from build123d import *

# Parameters (mm, degrees)
SKETCH1_W             = 80
SKETCH1_H             = 40
SKETCH1_R             = 2.25
BOSS_EXTRUDE1_DEPTH   = 5
BOSS_EXTRUDE1_2_DEPTH = 5
SKETCH2_W             = 80
SKETCH2_H             = 5
BOSS_EXTRUDE2_DEPTH   = 108.62
SKETCH3_W             = 43.85
SKETCH3_H             = 74
BOSS_EXTRUDE3_DEPTH   = 5
SKETCH5_W             = 29.85
SKETCH5_H             = 50
CUT_EXTRUDE2_DEPTH    = 10
CUT_EXTRUDE1_REACH    = 146.412
SKETCH4_R             = 1.3
FILLET1_R             = 3
FILLET2_R             = 3
SKETCH9_R             = 2.65
SKETCH9_R_2           = 1.05
BOSS_EXTRUDE5_DEPTH   = 4.75
SKETCH10_W            = 12
SKETCH10_H            = 6.8
CUT_EXTRUDE4_DEPTH    = 8
SKETCH11_W            = 80
SKETCH11_H            = 5
BOSS_EXTRUDE6_DEPTH   = 8
CUT_EXTRUDE5_REACH    = 167.987


with BuildPart() as part:
    # Sketch1 → Boss-Extrude1 (new body)
    with BuildSketch(Plane(origin=(0, 0, 0), x_dir=(1, 0, 0), z_dir=(0, 1, 0))):
        with Locations((0, 52)):
            Rectangle(SKETCH1_W, SKETCH1_H)
        with Locations(Location((-30.625, 53.044055982, 0), (0, 0, 270))):
            Circle(SKETCH1_R, mode=Mode.SUBTRACT)
        with Locations(Location((30.625, 53.044055982, 0), (0, 0, 90))):
            Circle(SKETCH1_R, mode=Mode.SUBTRACT)
    extrude(amount=BOSS_EXTRUDE1_DEPTH)



with BuildPart() as body_2:
    # Sketch1 → Boss-Extrude1 2 (new body)
    with BuildSketch(Plane(origin=(0, 0, 0), x_dir=(1, 0, 0), z_dir=(0, 1, 0))):
        with Locations((0, -52)):
            Rectangle(SKETCH1_W, SKETCH1_H)
        with Locations(Location((30.625, -53.044055982, 0), (0, 0, 270))):
            Circle(SKETCH1_R, mode=Mode.SUBTRACT)
        with Locations(Location((-30.625, -53.044055982, 0), (0, 0, 90))):
            Circle(SKETCH1_R, mode=Mode.SUBTRACT)
    extrude(amount=BOSS_EXTRUDE1_2_DEPTH)


with BuildPart() as part_1:
    add(part.part)

    add(body_2.part)  # Boss-Extrude2 merges body 2
    # Sketch2 → Boss-Extrude2 (add)
    with BuildSketch(Plane(origin=(0, 5, 0), x_dir=(1, 0, 0), z_dir=(0, 1, 0))):
        with Locations((0, 34.5)):
            Rectangle(SKETCH2_W, SKETCH2_H)
        with Locations((0, -34.5)):
            Rectangle(SKETCH2_W, SKETCH2_H)
    extrude(amount=BOSS_EXTRUDE2_DEPTH)

    # Sketch3 → Boss-Extrude3 (add)
    with BuildSketch(Plane(origin=(0, 113.62, 0), x_dir=(1, 0, 0), z_dir=(0, 1, 0))):
        with Locations((-3.925, 0)):
            Rectangle(SKETCH3_W, SKETCH3_H)
    extrude(amount=BOSS_EXTRUDE3_DEPTH)

    # Sketch5 → Cut-Extrude2 (cut)
    with BuildSketch(Plane.XZ.offset(-113.62)):
        with Locations((-3.925, 0)):
            Rectangle(SKETCH5_W, SKETCH5_H)
    extrude(amount=-CUT_EXTRUDE2_DEPTH, mode=Mode.SUBTRACT)

    # Sketch4 → Cut-Extrude1 (cut, up to next)
    with BuildSketch(Plane(origin=(0, 118.62, 0), x_dir=(1, 0, 0), z_dir=(0, 1, 0)), mode=Mode.PRIVATE) as cut_extrude1_sk1:
        with Locations(Location((-23, 20, 0), (0, 0, 270))):
            Circle(SKETCH4_R)
    cut_extrude1_tool1 = extrude(cut_extrude1_sk1.sketch, amount=-CUT_EXTRUDE1_REACH, mode=Mode.PRIVATE) & part_1.part
    # Sketch4 → Cut-Extrude1 (cut, up to next)
    with BuildSketch(Plane(origin=(0, 118.62, 0), x_dir=(1, 0, 0), z_dir=(0, 1, 0)), mode=Mode.PRIVATE) as cut_extrude1_sk2:
        with Locations(Location((15, 20, 0), (0, 0, 270))):
            Circle(SKETCH4_R)
    cut_extrude1_tool2 = extrude(cut_extrude1_sk2.sketch, amount=-CUT_EXTRUDE1_REACH, mode=Mode.PRIVATE) & part_1.part
    # Sketch4 → Cut-Extrude1 (cut, up to next)
    with BuildSketch(Plane(origin=(0, 118.62, 0), x_dir=(1, 0, 0), z_dir=(0, 1, 0)), mode=Mode.PRIVATE) as cut_extrude1_sk3:
        with Locations(Location((15, -20, 0), (0, 0, 270))):
            Circle(SKETCH4_R)
    cut_extrude1_tool3 = extrude(cut_extrude1_sk3.sketch, amount=-CUT_EXTRUDE1_REACH, mode=Mode.PRIVATE) & part_1.part
    # Sketch4 → Cut-Extrude1 (cut, up to next)
    with BuildSketch(Plane(origin=(0, 118.62, 0), x_dir=(1, 0, 0), z_dir=(0, 1, 0)), mode=Mode.PRIVATE) as cut_extrude1_sk4:
        with Locations(Location((-23, -20, 0), (0, 0, 270))):
            Circle(SKETCH4_R)
    cut_extrude1_tool4 = extrude(cut_extrude1_sk4.sketch, amount=-CUT_EXTRUDE1_REACH, mode=Mode.PRIVATE) & part_1.part
    add(cut_extrude1_tool1.solids().sort_by_distance((-23, 118.62, -20))[0], mode=Mode.SUBTRACT)
    add(cut_extrude1_tool2.solids().sort_by_distance((15, 118.62, -20))[0], mode=Mode.SUBTRACT)
    add(cut_extrude1_tool3.solids().sort_by_distance((15, 118.62, 20))[0], mode=Mode.SUBTRACT)
    add(cut_extrude1_tool4.solids().sort_by_distance((-23, 118.62, 20))[0], mode=Mode.SUBTRACT)

    # Fillet1
    fillet1_edges = [part_1.edges().sort_by_distance(p)[0] for p in [
        (0, 5, -37),
        (-3.925, 113.62, -32),
        (-3.925, 113.62, 32),
        (0, 5, 37),
    ]]
    fillet(fillet1_edges, radius=FILLET1_R)

    # Fillet2
    fillet2_edges = [part_1.edges().sort_by_distance(p)[0] for p in [
        (18, 113.62, -34.5),
        (-25.85, 113.62, -34.5),
        (-25.85, 113.62, 34.5),
        (18, 113.62, 34.5),
    ]]
    fillet(fillet2_edges, radius=FILLET2_R)

    # Sketch9 → Boss-Extrude5 (add)
    # profile 1 of 4: a face of its own
    with BuildSketch(Plane.XZ.offset(-113.62)):
        with Locations(Location((-23, 20, 0), (0, 0, 270))):
            Circle(SKETCH9_R)
        with Locations(Location((-23, 20, 0), (0, 0, 270))):
            Circle(SKETCH9_R_2, mode=Mode.SUBTRACT)
    # profile 2 of 4: a face of its own
    with BuildSketch(Plane.XZ.offset(-113.62)):
        with Locations(Location((-23, -20, 0), (0, 0, 270))):
            Circle(SKETCH9_R)
        with Locations(Location((-23, -20, 0), (0, 0, 270))):
            Circle(SKETCH9_R_2, mode=Mode.SUBTRACT)
    # profile 3 of 4: a face of its own
    with BuildSketch(Plane.XZ.offset(-113.62)):
        with Locations(Location((15, 20, 0), (0, 0, 270))):
            Circle(SKETCH9_R)
        with Locations(Location((15, 20, 0), (0, 0, 270))):
            Circle(SKETCH9_R_2, mode=Mode.SUBTRACT)
    # profile 4 of 4: a face of its own
    with BuildSketch(Plane.XZ.offset(-113.62)):
        with Locations(Location((15, -20, 0), (0, 0, 270))):
            Circle(SKETCH9_R)
        with Locations(Location((15, -20, 0), (0, 0, 270))):
            Circle(SKETCH9_R_2, mode=Mode.SUBTRACT)
    extrude(amount=BOSS_EXTRUDE5_DEPTH)

    # Sketch10 → Cut-Extrude4 (cut)
    with BuildSketch(Plane.XY.offset(37)):
        with Locations((6.7, 110.77)):
            Rectangle(SKETCH10_W, SKETCH10_H)
    extrude(amount=-CUT_EXTRUDE4_DEPTH, mode=Mode.SUBTRACT)

    # Sketch11 → Boss-Extrude6 (add)
    with BuildSketch(Plane(origin=(0, 0, 32), x_dir=(-1, 0, 0), z_dir=(0, 0, -1))):
        with Locations((0, 14.5)):
            Rectangle(SKETCH11_W, SKETCH11_H)
    extrude(amount=BOSS_EXTRUDE6_DEPTH)

    # Mirror3: part across plane


with BuildPart() as part_2:
    add(part_1.part)
    add(part_1.part.mirror(Plane.XY))

    # Sketch12 → Cut-Extrude5 (cut, up to next)
    with BuildSketch(Plane(origin=(0, 0, -37), x_dir=(-1, 0, 0), z_dir=(0, 0, -1)), mode=Mode.PRIVATE) as cut_extrude5_sk1:
        with BuildLine():
            Line((20, 31.025), (-20, 31.025))
            ThreePointArc((-20, 31.025), (-23, 34.025), (-20, 37.025))
            Line((-20, 37.025), (20, 37.025))
            ThreePointArc((20, 37.025), (23, 34.025), (20, 31.025))
        make_face()
    cut_extrude5_tool1 = extrude(cut_extrude5_sk1.sketch, amount=-CUT_EXTRUDE5_REACH, mode=Mode.PRIVATE) & part_2.part
    cut_extrude5 = cut_extrude5_tool1.solids().sort_by_distance((0, 34.025, -37))[0]
    add(cut_extrude5, mode=Mode.SUBTRACT)

    # Mirror4: Cut-Extrude5 across plane
    add(cut_extrude5.mirror(Plane.XY), mode=Mode.SUBTRACT)


solid = part_2.part
CAD build for the part. Positions are in the model's coordinates, mm. A direction names the side the tool comes from. Coordinates: 2 decimals unless noted, no trailing zeros. Loops run counter-clockwise (first coordinate to the right, second up) from the corner with the lowest first, then second, coordinate; pieces in that order, holes last. Notation, with made-up numbers: (67.25, 16) -> (126.25, 16) arc R19 ccw to (126.25, 43) -> close; hole circle Ø4 at (19.25, -13.5). An arc over 180 degrees is marked (long way). One line per item, written item: value.
1. Which spindle directions (+Z, -Z, +X, -X, +Y, -Y) get a long thin tool onto all of the face, cutting with end or side? Do faces 1 (the face through (-1, 5, 56)), 2 (the face through (18, 116, 1)), 3 (the face through (0, 31.025, 35)), 4 (the face through (13.99, 111.28, 17.55)), 5 (the face through (-1, 6, 32)). Say none if no direction does.
Answers:
face 1: +Z, +X, -X, +Y
face 2: +X, +Y
face 3: +Z, -Z
face 4: -Y
face 5: +X, -X, -Y
2. Flat gauge pins, fed straight in: P1, Ø10, axis at x = -28, y = 80, coming from the +Z side; P2, Ø10, axis at y = 13, z = 45, coming from the -X side; P3, Ø2.5, axis at x = -22.5, z = -20, coming from the -Y side; P4, Ø8, axis at x = -24, z = -42.5, coming from the +Y side. Where does each tip first touch, or does it go through?
Answers:
P1: stops at z = 37
P2: passes through
P3: stops at y = 108.87
P4: stops at y = 5.4
3. Drill centre lines: line 1 (X direction, y = 110.4, z = 20); line 2 (Z direction, x = 0, y = 48); line 3 (X direction, y = 117.4, z = 20). Where is each one in solid material? Low to high. Write a range as [from, to].
Answers:
line 1: x = [-25.65, -24.05], [-21.95, -20.35], [12.35, 13.95], [16.05, 17.65]
line 2: z = [-37, -32], [32, 37]
line 3: x = [-25.85, -24.3], [-21.7, -18.85], [11, 13.7], [16.3, 18]
4. Slice it at C-C on x = -15.5. Give the number of separate pieces and of enclosed holes in the cut face, and give its area (3 significant figures).
Answers:
separate pieces: 4
enclosed holes: 0
area: 1,630 mm^2
5. Slice it at D-D on z = -62. Write the cut outline in (x, y), and give its area (3 significant figures).
Answers:
outline: (-40, 0) -> (40, 0) -> (40, 5) -> (-40, 5) -> close
area: 400 mm^2
6. Pull direction X, two halves, no side cores. Call faces 6 (the face through (40, 40, -35)), 7 (the face through (23, 34, 35)), 8 (the face through (-25.85, 116, 1)), 9 (the face through (1, 12, 28)): pulls with the +X half, pulls with the -X half, needs draft (parallel to the pull), parting line crosses it, or undercut.
Answers:
face 6: pulls with the +X half
face 7: undercut
face 8: pulls with the -X half
face 9: needs draft
7. Slice it at B-B on z = 34.5. Write the cut outline in (x, y) (3 decimals).
Answers:
outline: (-40, 0) -> (40, 0) -> (40, 113.62) -> (21, 113.62) arc R3 cw to (18, 116.62) -> (18, 118.62) -> (-25.85, 118.62) -> (-25.85, 116.62) arc R3 cw to (-28.85, 113.62) -> (-40, 113.62) -> close; hole (-20, 31.025) -> (20, 31.025) arc R3 ccw to (20, 37.025) -> (-20, 37.025) arc R3 ccw to start
8. Slice it at A-A on y = 79.5. Write the cut outline in (x, z), and give its area (3 significant figures).
Answers:
outline: (-40, -37) -> (40, -37) -> (40, -32) -> (-40, -32) -> close; (-40, 32) -> (40, 32) -> (40, 37) -> (-40, 37) -> close
area: 800 mm^2
